Design review of the part built by this model. Coordinates are the model's own, in mm. A direction names the side the tool comes from. Round coordinates to 2 decimals unless told otherwise and drop trailing zeros. Write each loop counter-clockwise with the first axis right and the second up, starting at its lowest first coordinate (ties: lowest second). Pieces come first, ordered by that corner, then holes. Notation, with made-up numbers: (-13.75, 61.5) - (41.25, 61.5) arc R28 cw to (41.25, 84.5) - close; hole circle Ø7 at (-37, -13). An arc over 180 degrees is marked (long way). Use one line per item in the form item = value.
```python
from build123d import *

# Parameters (mm, degrees)
F0_R     = 51
F1_DEPTH = 3.5
F2_R     = 51
F2_R_2   = 48
F3_DEPTH = 16
F4_R     = 12.5
F5_DEPTH = 25
F6_SIZE  = 1
F7_SIZE  = 1


with BuildPart() as f1:
    # F0 (on Top) → F1 (new body)
    with BuildSketch(Plane.XY):
        Circle(F0_R)
    extrude(amount=F1_DEPTH)

    # F2 (on face) → F3 (join)
    with BuildSketch(Plane.XY.offset(3.5)):
        Circle(F2_R)
        Circle(F2_R_2, mode=Mode.SUBTRACT)
    extrude(amount=F3_DEPTH)

    # F4 (on face) → F5 (cut)
    with BuildSketch(Plane(origin=(0, 0, 0), x_dir=(1, 0, 0), z_dir=(0, 0, -1))):
        with Locations((0, 32)):
            Circle(F4_R)
        with Locations((0, -32)):
            Circle(F4_R)
    extrude(amount=-F5_DEPTH, mode=Mode.SUBTRACT)

    # F6
    f6_edges = [f1.edges().sort_by_distance(p)[0] for p in [
        (-51, 0, 0),
        (-12.5, 32, 0),
        (-12.5, -32, 0),
    ]]
    chamfer(f6_edges, length=F6_SIZE)

    # F7
    f7_edges = [f1.edges().sort_by_distance(p)[0] for p in [
        (-48, 0, 19.5),
    ]]
    chamfer(f7_edges, length=F7_SIZE)


solid = f1.part
```
Q1. For P1, Ø15, axis at x = 0, y = 32, coming from the -Z side; P2, Ø4, axis at x = -21.5, z = 15, coming from the -Y side; P3, Ø8, axis at y = -39, z = 7, coming from the -X side; P4, Ø1, axis at x = 31, y = -31.5, coming from the +Z side, all flat-tipped, find the tip position at first contact; note any pin that passes through.
Calculated:
P1 = through
P2 = -47.12
P3 = -37.09
P4 = 3.5
Q2. To check wall thickness, follow line 1 along Y through (x, z) = (0, 2.1); line 2 along Y through (x, z) = (-9.5, 1.25); line 3 along Z through (x, y) = (-8, -43.5). State the ranges of each line that lie inside material, in increasing order. Write a range as from..to.
Calculated:
line_1 = -51..-44.5, -19.5..19.5, 44.5..51
line_2 = -50.11..-40.12, -23.88..23.88, 40.12..50.11
line_3 = 0..3.5
Q3. Machinability: for faces 4 (the flat face through (-19, 46, 19.5)), 5 (the cylindrical face through (-47.954, 2.11, 10.895)), which of the approach directions +Z, -Z, +X, -X, +Y, -Y give a long, thin tool a straight path to every point of the face, cutting with its end or side? Answer none if there is none.
Calculated:
face_4 = +Z, +X, -X, +Y, -Y
face_5 = +Z
Q4. Draft analysis for pull direction Y (two halves, no side actions). For faces 1 (the cylindrical face through (6.72, 21.46, 2.23)), 2 (the cylindrical face through (-11.056, -49.787, 10.12)), 3 (the flat face through (-1, 1, 0)), state which applies: released by +Y, released by -Y, zero draft, split by the parting line, or undercut.
Calculated:
face_1 = undercut
face_2 = split by the parting line
face_3 = zero draft
Q5. We need section B-B on z = 10.25. Write out the cut boundary in (x, y), then the cut area to 3 significant figures.
Calculated:
outline = circle Ø102 at (0, 0); hole circle Ø96 at (0, 0)
area = 933 mm2
Q6. We need section A-A on x = 0. Write out the cut boundary in (y, z), then the cut area to 3 significant figures.
Calculated:
outline = (-51, 1) - (-50, 0) - (-45.5, 0) - (-44.5, 1) - (-44.5, 3.5) - (-48, 3.5) - (-48, 18.5) - (-49, 19.5) - (-51, 19.5) - close; (-19.5, 1) - (-18.5, 0) - (18.5, 0) - (19.5, 1) - (19.5, 3.5) - (-19.5, 3.5) - close; (44.5, 1) - (45.5, 0) - (50, 0) - (51, 1) - (51, 19.5) - (49, 19.5) - (48, 18.5) - (48, 3.5) - (44.5, 3.5) - close
area = 274 mm2
